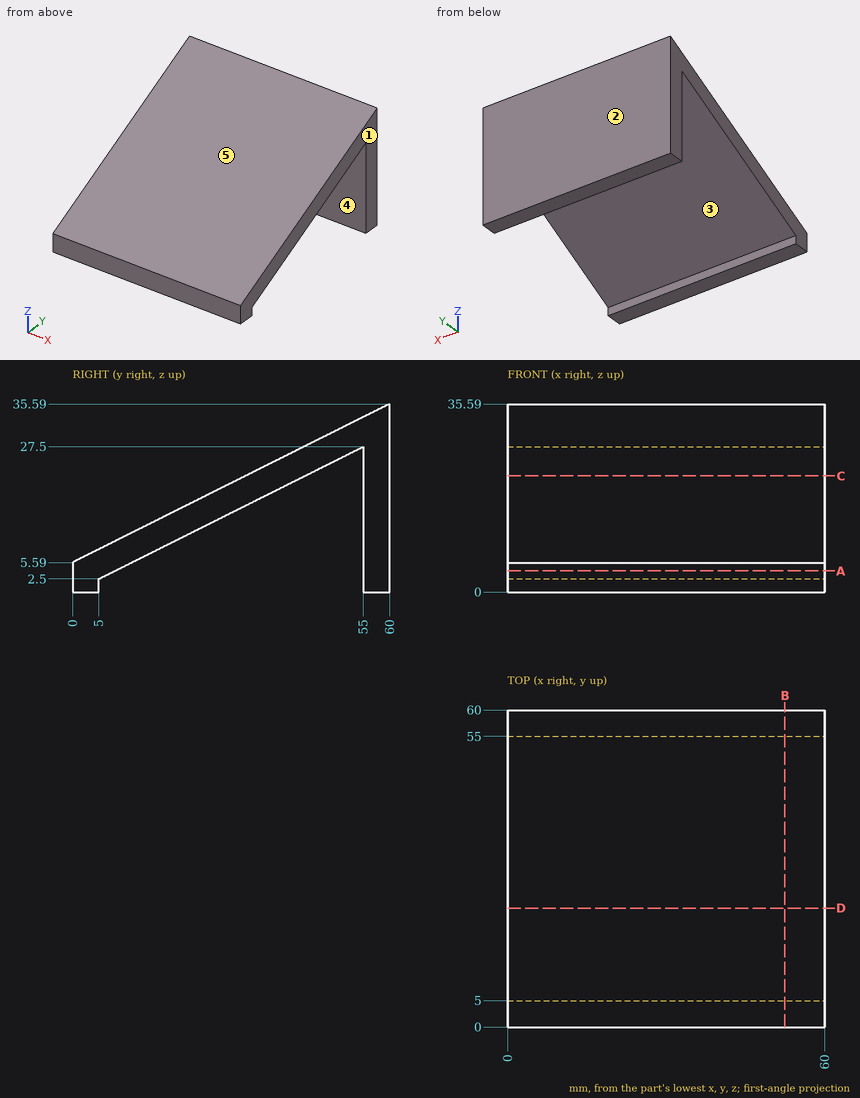
Input: dimensioned drawing with shaded views. Units: mm. Origin: part minimum x, y, z. A direction names the side the tool comes from. Round coordinates to 2 decimals unless told otherwise and drop trailing zeros. Order: outer loops, then holes, each group sorted by start corner. A loop starts at its lowest first (then second) coordinate and runs counter-clockwise, first axis right, second up. Notation, with made-up numbers: M 24,38.5 L 45,38.5 A13 cw 45,45.5 Z; hole C 23.25,-12.5 d6. An arc over 180 degrees is marked long. Use one line per item in the form item = value. Start each with the question number.
Q1. Cut plane B-B (x = 52.5). Return loops of the section in (y, z).
Q2. Cut plane D-D (y = 22.5). Return loops of the section in (x, z), and give its area (3 significant figures).
Q3. Material intervals for line 1 (Y direction, x = 55.5, z = 2); line 2 (Y direction, x = 3, z = 6); line 3 (Z direction, x = 39, y = 21), sorted ascending. Write a range as [from, to].
Q4. Pin query (flat end, axial travel): pin 1 Ø14 at (x, z) = (43.5, 10) entering from -Y; pin 2 Ø2 at (x, y) = (15.5, 43) entering from -Z; pin 3 Ø10 at (y, z) = (26, 4) entering from -X; pin 4 Ø6 at (x, y) = (32, 38.5) entering from -Z. Return the tip coordinate at first contact, or that it passes through.
Q5. Cut plane C-C (z = 22). Return loops of the section in (x, y), and give its area (3 significant figures).
Q6. Access query for the marked faces 4 and 5. Directions: +Z, -Z, +X, -X, +Y, -Y. A direction counts if a zero-diameter tool reaches every point of the face in a straight line with its end or side. Return the directions, or none.
Q7. Mould query, pull axis Y, two halves, no side actions, for the marked faces 1, 2 and 3. Classes: +Y half, -Y half, draft (parallel to the pull), parting line (faces both ways), or undercut.
Q8. Cut plane A-A (z = 4). Return loops of the section in (x, y), and give its area (3 significant figures).
Geometry results:
q1.outline = M 0,0 L 5,0 L 5,2.5 L 55,27.5 L 55,0 L 60,0 L 60,35.59 L 0,5.59 Z
q2.outline = M 0,11.25 L 60,11.25 L 60,16.84 L 0,16.84 Z
q2.area = 335 mm^2
q3.line_1 = [0, 5], [55, 60]
q3.line_2 = [0.82, 12], [55, 60]
q3.line_3 = [10.5, 16.09]
q4.pin_1 = 0
q4.pin_2 = 21
q4.pin_3 = through
q4.pin_4 = 17.75
q5.outline = M 0,32.82 L 60,32.82 L 60,44 L 0,44 Z; M 0,55 L 60,55 L 60,60 L 0,60 Z
q5.area = 971 mm^2
q6.face_4 = -Z, +X, -X
q6.face_5 = +Z, +X, -X, -Y
q7.face_1 = draft
q7.face_2 = +Y half
q7.face_3 = undercut
q8.outline = M 0,0 L 60,0 L 60,8 L 0,8 Z; M 0,55 L 60,55 L 60,60 L 0,60 Z
q8.area = 780 mm^2
